Here's how the part is built. I have some questions about the finished solid (model axes, mm). A direction names the side the tool comes from. Round coordinates to 2 decimals unless told otherwise and drop trailing zeros. Order: outer loops, then holes, each group sorted by start corner. A loop starts at its lowest first (then second) coordinate and runs counter-clockwise, first axis right, second up.
```python
from build123d import *

# Parameters (mm, degrees)
SKETCH1_W           = 76
SKETCH1_H           = 60
BOSS_EXTRUDE1_DEPTH = 4.5
CUT_EXTRUDE1_DEPTH  = 3
CUT_EXTRUDE2_DEPTH  = 49.507731343
FILLET1_R           = 5
SKETCH4_R           = 1.6
CUT_EXTRUDE3_DEPTH  = 49.623553963


with BuildPart() as part:
    # Sketch1 → Boss-Extrude1 (new body)
    with BuildSketch(Plane(origin=(0, 0, 0), x_dir=(1, 0, 0), z_dir=(0, 1, 0))):
        Rectangle(SKETCH1_W, SKETCH1_H)
    extrude(amount=BOSS_EXTRUDE1_DEPTH)

    # Sketch2 → Cut-Extrude1 (cut)
    with BuildSketch(Plane(origin=(0, 4.5, 0), x_dir=(1, 0, 0), z_dir=(0, 1, 0))):
        with BuildLine():
            Line((20, -5.9), (38, -5.9))
            Line((38, -5.9), (38, -22.1))
            Line((38, -22.1), (20, -22.1))
            ThreePointArc((20, -22.1), (11.9, -14), (20, -5.9))
        make_face()
    cut_extrude1 = extrude(amount=-CUT_EXTRUDE1_DEPTH, mode=Mode.SUBTRACT)

    # Sketch3 → Cut-Extrude2 (cut, through all)
    with BuildSketch(Plane(origin=(0, 1.5, 0), x_dir=(1, 0, 0), z_dir=(0, 1, 0))):
        with BuildLine():
            Line((20, -9.5), (33, -9.5))
            Line((33, -9.5), (38, -5.9))
            Line((38, -5.9), (38, -22.1))
            Line((38, -22.1), (33, -18.5))
            Line((33, -18.5), (20, -18.5))
            ThreePointArc((20, -18.5), (15.5, -14), (20, -9.5))
        make_face()
    cut_extrude2 = extrude(amount=-CUT_EXTRUDE2_DEPTH, mode=Mode.SUBTRACT)

    # Mirror1: Cut-Extrude1, Cut-Extrude2 across plane
    add(cut_extrude1.mirror(Plane(origin=(0, 0, 0), x_dir=(0, 0, 1), z_dir=(1, 0, 0))), mode=Mode.SUBTRACT)
    add(cut_extrude2.mirror(Plane(origin=(0, 0, 0), x_dir=(0, 0, 1), z_dir=(1, 0, 0))), mode=Mode.SUBTRACT)

    # Fillet1
    fillet1_edges = [part.edges().sort_by_distance(p)[0] for p in [
        (38, 2.25, 30),
        (-38, 2.25, 30),
        (-38, 2.25, -30),
        (38, 2.25, -30),
    ]]
    fillet(fillet1_edges, radius=FILLET1_R)

    # Sketch4 → Cut-Extrude3 (cut, through all)
    with BuildSketch(Plane(origin=(0, 4.5, 0), x_dir=(1, 0, 0), z_dir=(0, 1, 0))):
        with Locations(Location((-15, 25, 0), (0, 0, 270))):
            Circle(SKETCH4_R)
        with Locations(Location((15, 25, 0), (0, 0, 270))):
            Circle(SKETCH4_R)
        with Locations(Location((33, -25, 0), (0, 0, 270))):
            Circle(SKETCH4_R)
        with Locations(Location((-33, -25, 0), (0, 0, 270))):
            Circle(SKETCH4_R)
        with Locations(Location((0, -15, 0), (0, 0, 270))):
            Circle(SKETCH4_R)
    extrude(amount=-CUT_EXTRUDE3_DEPTH, mode=Mode.SUBTRACT)


solid = part.part
```
1. If we section it at A-A, the plane x = 0: Write out the boundary of the cut face in (y, z), and give its area (3 significant figures).
Evaluation:
outline: (0, -30) - (4.5, -30) - (4.5, 13.4) - (0, 13.4) - close; (0, 16.6) - (4.5, 16.6) - (4.5, 30) - (0, 30) - close
area: 256 mm2
2. If we section it at C-C, the plane x = -28: Write out the boundary of the cut face in (y, z), and give its area (3 significant figures).
Evaluation:
outline: (0, -30) - (4.5, -30) - (4.5, 5.9) - (1.5, 5.9) - (1.5, 9.5) - (0, 9.5) - close; (0, 18.5) - (1.5, 18.5) - (1.5, 22.1) - (4.5, 22.1) - (4.5, 30) - (0, 30) - close
area: 208 mm2
3. If we section it at B-B, the plane y = 0.75: Write out the boundary of the cut face in (x, z).
Evaluation:
outline: (-38, -25) arc R5 ccw to (-33, -30) - (33, -30) arc R5 ccw to (38, -25) - (38, 5.9) - (33, 9.5) - (20, 9.5) arc R4.5 cw to (20, 18.5) - (33, 18.5) - (38, 22.1) - (38, 25) arc R5 ccw to (33, 30) - (-33, 30) arc R5 ccw to (-38, 25) - (-38, 22.1) - (-33, 18.5) - (-20, 18.5) arc R4.5 cw to (-20, 9.5) - (-33, 9.5) - (-38, 5.9) - close; hole circle Ø3.2 at (-33, 25); hole circle Ø3.2 at (-15, -25); hole circle Ø3.2 at (0, 15); hole circle Ø3.2 at (15, -25); hole circle Ø3.2 at (33, 25)
4. I need wall thicknesses on probe 1 along X at (y, z) = (1.3, 25); probe 2 along Z at (x, y) = (15.5, 1.6); probe 3 along Z at (x, y) = (23.5, 0.5). Which ranges of each line are inside material? Lowest first, please.
Evaluation:
probe 1: x = -38 to -34.6, -31.4 to 31.4, 34.6 to 38
probe 2: z = -30 to -26.52, -23.48 to 7.27, 20.73 to 30
probe 3: z = -30 to 9.5, 18.5 to 30
5. I'm going to push flat-ended pins straight in: P1, Ø8, axis at x = 27.5, z = 11.5, coming from the +Y side; P2, Ø3, axis at x = 15, z = -25, coming from the -Y side. Where does each tip first touch, or does it pass through?
Evaluation:
P1: stops at y = 1.5
P2: passes through
6. On a 3-axis mill with a long thin cutter (end or side, diameter ignored), from which of +Z, -Z, +X, -X, +Y, -Y can I reach the whole of each face in a straight line? I mean faces 1 (the flat face through (35.5, 0.8, 20.3)), 2 (the flat face through (-26, 1, 9.5)), 3 (the cylindrical face through (-11.9, 3.02, 14.18)), 4 (the flat face through (29, 3, 5.9)). Say none if no direction works.
Evaluation:
face 1: +X, +Y, -Y
face 2: -X, +Y, -Y
face 3: -X, +Y
face 4: +X, +Y
7. If we mould it in two halves opening along Z, with no side actions, what happens to faces 5 (the flat face through (-38, 2, -9)), 6 (the flat face through (-35.5, 0.8, 7.7)), 7 (the flat face through (0, 2, 30))? For each: released by +Z, released by -Z, zero draft, split by the parting line, or undercut.
Evaluation:
face 5: zero draft
face 6: undercut
face 7: released by +Z
